Geometry: final body of the model. Coordinates: model frame, mm. Give positions to 0.01 mm unless a question says otherwise; leave off trailing zeros. Loops run counter-clockwise (first coordinate to the right, second up) from the corner with the lowest first, then second, coordinate; pieces in that order, holes last.
from build123d import *

# Parameters (mm, degrees)
ESQUISSE1_R             = 2.05
BOSS_EXTRU_1_DEPTH      = 9.75
BOSS_EXTRU_2_DEPTH      = 5
BOSS_EXTRU_2_DEPTH_BACK = 15
ESQUISSE2_R             = 5
ESQUISSE2_R_2           = 2.05


with BuildPart() as part:
    # Esquisse1 → Boss.-Extru.1 (new body)
    with BuildSketch(Plane(origin=(0, 0, 0), x_dir=(1, 0, 0), z_dir=(0, 1, 0))):
        with BuildLine():
            Line((-5, 0), (-5, 60))
            ThreePointArc((-5, 60), (0, 65), (5, 60))
            Line((5, 60), (5, 0))
            ThreePointArc((5, 0), (0, -5), (-5, 0))
        make_face()
        with Locations(Location((0, 60, 0), (0, 0, 270))):
            Circle(ESQUISSE1_R, mode=Mode.SUBTRACT)
        with Locations(Location((0, 0, 0), (0, 0, 270))):
            Circle(ESQUISSE1_R, mode=Mode.SUBTRACT)
    extrude(amount=BOSS_EXTRU_1_DEPTH)

    # Esquisse2 → Boss.-Extru.2 (add, two sides: drawn at the far end of the back side and taken through both)
    with BuildSketch(Plane(origin=(0, 9.75, 0), x_dir=(1, 0, 0), z_dir=(0, 1, 0)).offset(-BOSS_EXTRU_2_DEPTH_BACK)):
        with Locations(Location((0, 60, 0), (0, 0, 270))):
            Circle(ESQUISSE2_R)
        with Locations(Location((0, 60, 0), (0, 0, 270))):
            Circle(ESQUISSE2_R_2, mode=Mode.SUBTRACT)
    extrude(amount=BOSS_EXTRU_2_DEPTH + BOSS_EXTRU_2_DEPTH_BACK)


solid = part.part
Item 1: Section query A-A on x = 0. Return loops of the section in (y, z).
Values follow:
outline: (-5.25, -65) - (14.75, -65) - (14.75, -62.05) - (-5.25, -62.05) - close; (-5.25, -57.95) - (14.75, -57.95) - (14.75, -55) - (9.75, -55) - (9.75, -2.05) - (0, -2.05) - (0, -55) - (-5.25, -55) - close; (0, 2.05) - (9.75, 2.05) - (9.75, 5) - (0, 5) - close
Item 2: Section query D-D on z = -19. Return loops of the section in (x, y).
Values follow:
outline: (-5, 0) - (5, 0) - (5, 9.75) - (-5, 9.75) - close
Item 3: Section query C-C on x = -4. Return loops of the section in (y, z).
Values follow:
outline: (-5.25, -63) - (14.75, -63) - (14.75, -57) - (9.75, -57) - (9.75, 3) - (0, 3) - (0, -57) - (-5.25, -57) - close
Item 4: Ray query, probe 1 along X at (y, z) = (2, -60); probe 2 along Z at (x, y) = (-0.75, 9.25); probe 3 along Y at (x, z) = (-4.25, -7.5). Return the intervals inside material, ascending.
Values follow:
probe 1: x = -5 to -2.05, 2.05 to 5
probe 2: z = -64.94 to -61.91, -58.09 to -1.91, 1.91 to 4.94
probe 3: y = 0 to 9.75
Item 5: Pin query (flat end, axial travel): pin 1 (5 mm diameter, centred on x = -3, y = 12, fed in from +Z); pin 2 (1 mm diameter, centred on x = 4, z = -24, fed in from -Y); pin 3 (6 mm diameter, centred on x = -4, y = 4, fed in from +Z). Return the tip coordinate at first contact, or that it passes through.
Values follow:
pin 1: stops at z = 4.62
pin 2: stops at y = 0
pin 3: stops at z = 4.9
Item 6: Section query B-B on y = 6.5. Return loops of the section in (x, z).
Values follow:
outline: (-5, -60) arc R5 ccw to (5, -60) - (5, 0) arc R5 ccw to (-5, 0) - close; hole circle Ø4.1 at (0, -60); hole circle Ø4.1 at (0, 0)
Item 7: Draft query along Z for faces 1 (the face through (0, 5, -65)), 2 (the face through (0.1, -5.25, -57.8)), 3 (the face through (2.033, 4.807, -0.267)), 4 (the face through (0.09, 4.61, -62.05)). Return one class per face: +Z half, -Z half, draft (parallel to the pull), parting line (faces both ways), or undercut.
Values follow:
face 1: parting line
face 2: draft
face 3: undercut
face 4: undercut
